```python
from build123d import *

# Parameters (mm, degrees)
F0_W     = 80
F0_H     = 50
F1_DEPTH = 15
F2_W     = 31.118957
F2_H     = 16.829639
F3_DEPTH = 40
F4_R     = 5
F5_DEPTH = 34.441523


with BuildPart() as f1:
    # F0 (on Top) → F1 (new body)
    with BuildSketch(Plane.XY):
        with Locations((40, 25)):
            Rectangle(F0_W, F0_H)
    extrude(amount=F1_DEPTH)

    # F2 (on face) → F3 (join)
    with BuildSketch(Plane.XY.offset(15)):
        with Locations((40.604838, 23.974297)):
            Rectangle(F2_W, F2_H)
    extrude(amount=F3_DEPTH)

    # F4 (on face) → F5 (cut, through all)
    with BuildSketch(Plane.XZ.offset(-15.559477)):
        with Locations((39.652213, 41.597784)):
            Circle(F4_R)
    extrude(amount=-F5_DEPTH, mode=Mode.SUBTRACT)


solid = f1.part
```
Could you check a few things on this model? Use its own coordinates, in mm. A direction names the side the tool comes from. Coordinates: 2 decimals unless noted, no trailing zeros. Order: outer loops, then holes, each group sorted by start corner. A loop starts at its lowest first (then second) coordinate and runs counter-clockwise, first axis right, second up. Notation, with made-up numbers: M 22,74.25 L 31,74.25 A25 ccw 31,107.25 Z; hole C -21.75,-14 d2. An arc over 180 degrees is marked long. Use a Markdown table: item, result. Add a question column.
Q1. I'm going to push flat-ended pins straight in: pin 1 (13 mm diameter, centred on x = 39.65, z = 41.6, fed in from -Y); pin 2 (9.5 mm diameter, centred on x = 42, z = 28.5, fed in from +Y); pin 3 (13.5 mm diameter, centred on y = 27, z = 32.5, fed in from -X); pin 4 (5 mm diameter, centred on y = 11.5, z = 26.5, fed in from -X). Where does each tip first touch, or does it pass through?
Q2. Which directions (+Z, -Z, +X, -X, +Y, -Y) give clear straight access to the entire face, cutting with the end or side of a thin tool? Please do faces 1 (the flat face through (25.045, 24, 35)), 2 (the flat face through (56.164, 24, 35)), 3 (the flat face through (40, 15.559, 35)).
Q3. We'd pull the mould along Z, two halves only. Please class faces 4 (the cylindrical face through (35.68, 23.86, 38.56)), 5 (the flat face through (39, 50, 7)), 6 (the flat face through (39, 25, 0)): pulls with the +Z half, pulls with the -Z half, needs draft (parallel to the pull), parting line crosses it, or undercut.
Q4. I want a section at B-B on x = 42. List the corners of the cut face in (y, z) for me.
Q5. If I drill on L1, parallel to Z at x = 59, y = 25; L2, parallel to X at y = 30.5, z = 52.5; L3, parallel to X at y = 23.5, z = 40, over which ranges is the centre line in solid material (lowest first)?
Q6. I want a section at C-C on y = 17. List the corners of the cut face in (x, z) for me, then the cut area to 3 significant figures.
Q7. I want a section at A-A on z = 45. List the corners of the cut face in (x, y) for me.
Q8. I want a section at D-D on x = 54. List the corners of the cut face in (y, z) for me.
Checked values:
| question | item | result |
|---|---|---|
| 1 | pin 1 | y = 15.56 |
| 1 | pin 2 | y = 32.39 |
| 1 | pin 3 | x = 25.05 |
| 1 | pin 4 | through |
| 2 | face 1 | +Z, -X, +Y, -Y |
| 2 | face 2 | +Z, +X, +Y, -Y |
| 2 | face 3 | +Z, +X, -X, -Y |
| 3 | face 4 | undercut |
| 3 | face 5 | needs draft |
| 3 | face 6 | pulls with the -Z half |
| 4 | outline | M 0,0 L 50,0 L 50,15 L 32.39,15 L 32.39,37.18 L 15.56,37.18 L 15.56,15 L 0,15 Z; M 15.56,46.01 L 32.39,46.01 L 32.39,55 L 15.56,55 Z |
| 5 | L1 | 0 to 15 |
| 5 | L2 | 25.05 to 56.16 |
| 5 | L3 | 25.05 to 34.91, 44.39 to 56.16 |
| 6 | outline | M 0,0 L 80,0 L 80,15 L 56.16,15 L 56.16,55 L 25.05,55 L 25.05,15 L 0,15 Z; hole C 39.65,41.6 d10 |
| 6 | area | 2,370 mm² |
| 7 | outline | M 25.05,15.56 L 35.99,15.56 L 35.99,32.39 L 25.05,32.39 Z; M 43.32,15.56 L 56.16,15.56 L 56.16,32.39 L 43.32,32.39 Z |
| 8 | outline | M 0,0 L 50,0 L 50,15 L 32.39,15 L 32.39,55 L 15.56,55 L 15.56,15 L 0,15 Z |
